Autodesk Inventor part; units mm, degrees
ref_plane "side_4d_XY" through (-20, 0, -272.5) normal (-1, 0, 0) x (0, 1, 0)
ref_plane "side_4d_YZ" through (-20, 0, -272.5) normal (0, 1, 0) x (0, 0, -1)
ref_plane "side_4d_ZX" through (-20, 0, -272.5) normal (0, 0, -1) x (-1, 0, 0)
sketch "Skizze_1" plane through (0, 0, 0) normal (0, 0, 1) x (1, 0, 0)
  arc A0 (-20, -17) -> (-17, -20) centre (-17, -17) ccw
  line L0 (-17, -20) -> (-4.1, -20)
  line L1 (-4.1, -20) -> (-4.1, -17)
  line L2 (-4.1, -17) -> (-10.5, -17)
  line L3 (-10.5, -17) -> (-10.5, -13.6627)
  arc A1 (-10.0314, -12.5314) -> (-10.5, -13.6627) centre (-8.9002, -13.6627) ccw
  line L4 (-10.0314, -12.5314) -> (-7.4645, -9.9645)
  arc A2 (-3.9289, -8.5) -> (-7.4645, -9.9645) centre (-3.9289, -13.5) ccw
  line L5 (-3.9289, -8.5) -> (3.9289, -8.5)
  arc A3 (7.4645, -9.9645) -> (3.9289, -8.5) centre (3.9289, -13.5) ccw
  line L6 (7.4645, -9.9645) -> (10.0314, -12.5314)
  arc A4 (10.5, -13.6627) -> (10.0314, -12.5314) centre (8.9002, -13.6627) ccw
  line L7 (10.5, -13.6627) -> (10.5, -17)
  line L8 (10.5, -17) -> (4.1, -17)
  line L9 (4.1, -17) -> (4.1, -20)
  line L10 (4.1, -20) -> (17, -20)
  arc A5 (17, -20) -> (20, -17) centre (17, -17) ccw
  line L11 (20, -17) -> (20, -4.1)
  line L12 (20, -4.1) -> (17, -4.1)
  line L13 (17, -4.1) -> (17, -10.5)
  line L14 (17, -10.5) -> (13.6627, -10.5)
  arc A6 (12.5314, -10.0314) -> (13.6627, -10.5) centre (13.6627, -8.9002) ccw
  line L15 (12.5314, -10.0314) -> (9.9645, -7.4645)
  arc A7 (8.5, -3.9289) -> (9.9645, -7.4645) centre (13.5, -3.9289) ccw
  line L16 (8.5, -3.9289) -> (8.5, 3.9289)
  arc A8 (9.9645, 7.4645) -> (8.5, 3.9289) centre (13.5, 3.9289) ccw
  line L17 (9.9645, 7.4645) -> (12.5314, 10.0314)
  arc A9 (13.6627, 10.5) -> (12.5314, 10.0314) centre (13.6627, 8.9002) ccw
  line L18 (13.6627, 10.5) -> (17, 10.5)
  line L19 (17, 10.5) -> (17, 4.1)
  line L20 (17, 4.1) -> (20, 4.1)
  line L21 (20, 4.1) -> (20, 17)
  arc A10 (20, 17) -> (17, 20) centre (17, 17) ccw
  line L22 (17, 20) -> (4.1, 20)
  line L23 (4.1, 20) -> (4.1, 17)
  line L24 (4.1, 17) -> (10.5, 17)
  line L25 (10.5, 17) -> (10.5, 13.6627)
  arc A11 (10.0314, 12.5314) -> (10.5, 13.6627) centre (8.9002, 13.6627) ccw
  line L26 (10.0314, 12.5314) -> (7.4645, 9.9645)
  arc A12 (3.9289, 8.5) -> (7.4645, 9.9645) centre (3.9289, 13.5) ccw
  line L27 (3.9289, 8.5) -> (-3.9289, 8.5)
  arc A13 (-7.4645, 9.9645) -> (-3.9289, 8.5) centre (-3.9289, 13.5) ccw
  line L28 (-7.4645, 9.9645) -> (-10.0314, 12.5314)
  arc A14 (-10.5, 13.6627) -> (-10.0314, 12.5314) centre (-8.9002, 13.6627) ccw
  line L29 (-10.5, 13.6627) -> (-10.5, 17)
  line L30 (-10.5, 17) -> (-4.1, 17)
  line L31 (-4.1, 17) -> (-4.1, 20)
  line L32 (-4.1, 20) -> (-17, 20)
  arc A15 (-17, 20) -> (-20, 17) centre (-17, 17) ccw
  line L33 (-20, 17) -> (-20, 4.1)
  line L34 (-20, 4.1) -> (-17, 4.1)
  line L35 (-17, 4.1) -> (-17, 10.5)
  line L36 (-17, 10.5) -> (-13.6627, 10.5)
  arc A16 (-12.5314, 10.0314) -> (-13.6627, 10.5) centre (-13.6627, 8.9002) ccw
  line L37 (-12.5314, 10.0314) -> (-9.9645, 7.4645)
  arc A17 (-8.5, 3.9289) -> (-9.9645, 7.4645) centre (-13.5, 3.9289) ccw
  line L38 (-8.5, 3.9289) -> (-8.5, -3.9289)
  arc A18 (-9.9645, -7.4645) -> (-8.5, -3.9289) centre (-13.5, -3.9289) ccw
  line L39 (-9.9645, -7.4645) -> (-12.5314, -10.0314)
  arc A19 (-13.6627, -10.5) -> (-12.5314, -10.0314) centre (-13.6627, -8.9002) ccw
  line L40 (-13.6627, -10.5) -> (-17, -10.5)
  line L41 (-17, -10.5) -> (-17, -4.1)
  line L42 (-17, -4.1) -> (-20, -4.1)
  line L43 (-20, -4.1) -> (-20, -17)
  circle A20 centre (0, 0) radius 6
extrude "Extrusion1" add sketch "Skizze_1" against normal blind 545
sketch "Sketch2" plane through (0, 0, 0) normal (0, 0, 1) x (1, 0, 0)
  point P0 (-15, -15)
hole "Drilling 1" at (-15, -15, 0) direction (0, 0, -1) diameter 5 depth 6000
sketch "Sketch3" plane through (0, 0, 0) normal (0, 0, 1) x (1, 0, 0)
  point P0 (15, -15)
hole "Drilling 2" at (15, -15, 0) direction (0, 0, -1) diameter 5 depth 6000
sketch "Sketch4" plane through (0, 0, 0) normal (0, 0, 1) x (1, 0, 0)
  point P0 (15, 15)
hole "Drilling 3" at (15, 15, 0) direction (0, 0, -1) diameter 5 depth 6000
sketch "Sketch5" plane through (0, 0, 0) normal (0, 0, 1) x (1, 0, 0)
  point P0 (-15, 15)
hole "Drilling 4" at (-15, 15, 0) direction (0, 0, -1) diameter 5 depth 6000
ref_plane "side_4d_XY" through (-20, 0, -272.5) normal (-1, 0, 0) x (0, 1, 0)
ref_plane "side_4d_YZ" through (-20, 0, -272.5) normal (0, 1, 0) x (0, 0, -1)
ref_plane "side_4d_ZX" through (-20, 0, -272.5) normal (0, 0, -1) x (-1, 0, 0)
ref_plane "side_1a_XY" through (0, 20, -272.5) normal (0, 1, 0) x (1, 0, 0)
ref_plane "side_1a_YZ" through (0, 20, -272.5) normal (1, 0, 0) x (0, 0, -1)
ref_plane "side_1a_ZX" through (0, 20, -272.5) normal (0, 0, -1) x (0, 1, 0)
ref_plane "side_2b_XY" through (20, 0, -272.5) normal (1, 0, 0) x (0, -1, 0)
ref_plane "side_2b_YZ" through (20, 0, -272.5) normal (0, -1, 0) x (0, 0, -1)
ref_plane "side_2b_ZX" through (20, 0, -272.5) normal (0, 0, -1) x (1, 0, 0)
ref_plane "side_3c_XY" through (0, -20, -272.5) normal (0, -1, 0) x (-1, 0, 0)
ref_plane "side_3c_YZ" through (0, -20, -272.5) normal (-1, 0, 0) x (0, 0, -1)
ref_plane "side_3c_ZX" through (0, -20, -272.5) normal (0, 0, -1) x (0, -1, 0)
ref_plane "end_XY" through (0, 0, -545) normal (0, 0, -1) x (1, 0, 0)
ref_plane "end_YZ" through (0, 0, -545) normal (1, 0, 0) x (0, -1, 0)
ref_plane "end_ZX" through (0, 0, -545) normal (0, -1, 0) x (0, 0, -1)
ref_plane "start_XY" through (0, 0, 0) normal (0, 0, 1) x (1, 0, 0)
ref_plane "start_YZ" through (0, 0, 0) normal (1, 0, 0) x (0, 1, 0)
ref_plane "start_ZX" through (0, 0, 0) normal (0, 1, 0) x (0, 0, 1)
properties part number "MayTec 1.11.040040.43S_Profile 40x40, 4E, S_545_Detail_(0;0,0,0)"
Could you check a few things on this model? Use its own coordinates, in mm. Round coordinates to 2 decimals unless told otherwise and drop trailing zeros. Use CSV: the item, a comma, the result in double quotes.
Item 1: If we section it at A-A on z = -466.5: Count the separate pieces of the cut face and the enclosed holes in it, then the cut area to 3 significant figures.
Here are the results:
separate pieces,"1"
enclosed holes,"5"
area,"674 mm²"
Item 2: Will these pins go through, and if not, where does the flat tip stop? pin 1 (6 mm diameter, centred on x = -6, y = -10.5, fed in from -Z); pin 2 (0.9 mm diameter, centred on x = -18, z = -233, fed in from -Y); pin 3 (1.5 mm diameter, centred on y = -19, z = -272, fed in from -X); pin 4 (1.5 mm diameter, centred on x = -19, z = -194.5, fed in from +Y).
Here are the results:
pin 1,"stops at z = -545"
pin 2,"stops at y = -19.95"
pin 3,"stops at x = -19.73"
pin 4,"stops at y = 19.73"
Item 3: I need wall thicknesses on L1, parallel to X at y = 15, z = -397.5; L2, parallel to X at y = 15.5, z = -446.5. Which ranges of each line are inside material? Lowest first, please. Write a range as [from, to].
Here are the results:
L1,"x = [-20, -17.5], [-12.5, -10.5], [10.5, 12.5], [17.5, 20]"
L2,"x = [-20, -17.45], [-12.55, -10.5], [10.5, 12.55], [17.45, 20]"
Item 4: If we mould it in two halves opening along Y, with no side actions, what happens to faces 1 (the cylindrical face through (-6, 0, -269)), 2 (the flat face through (-5, -4, -545)), 3 (the flat face through (11, 20, -269))? For each: pulls with the +Y half, pulls with the -Y half, needs draft (parallel to the pull), parting line crosses it, or undercut.
Here are the results:
face 1,"undercut"
face 2,"needs draft"
face 3,"pulls with the +Y half"
